Autodesk Fusion 360 part; units mm, degrees
sketch "Sketch1" plane through (0, 0, 0) normal (0, 0, 1) x (1, 0, 0)
  line L0 (19.05, -25.4) -> (-19.05, -25.4)
  line L1 (-19.05, -25.4) -> (-19.05, 25.4)
  line L2 (-19.05, 25.4) -> (19.05, 25.4)
  line L3 (19.05, 25.4) -> (19.05, -25.4)
  line L4 (19.05, -25.4) -> (-19.05, 25.4) construction
  line L5 (-19.05, -25.4) -> (19.05, 25.4) construction
  dimension "d1" = 38.1
  dimension "d2" = 50.8
extrude "Extrude1" add sketch "Sketch1" along normal blind 6.35
sketch "Sketch2" plane through (0, 0, 6.35) normal (0, 0, 1) x (-1, 0, 0)
  line L0 (-19.05, -25.4) -> (19.05, -25.4)
  line L1 (19.05, -25.4) -> (19.05, 25.4)
  line L2 (19.05, 25.4) -> (-19.05, 25.4)
  line L3 (-19.05, 25.4) -> (-19.05, -25.4)
  line L4 (19.05, -12.7) -> (3.81, -12.7)
  line L5 (3.81, -12.7) -> (3.81, 12.7)
  line L6 (3.81, 12.7) -> (19.05, 12.7)
  line L7 (19.05, 12.7) -> (19.05, -12.7)
  line L8 (-19.05, -15.24) -> (3.81, -15.24)
  line L9 (3.81, -15.24) -> (3.81, 15.24)
  line L10 (3.81, 15.24) -> (-19.05, 15.24)
  line L11 (-19.05, 15.24) -> (-19.05, -15.24)
  dimension "d5" = 15.24
  dimension "d6" = 25.4
  dimension "d7" = 12.7
  dimension "d9" = 10.16
  dimension "d14" = 10.16
extrude "Extrude2" add sketch "Sketch2" along normal blind 15.24 contours L1 L4 L5 L6 L7 L9
extrude "Extrude3" add sketch "Sketch2" along normal blind 29.21 contours L3 L5 L8 L9 L10 L11
sketch "Sketch3" plane through (0, -12.7, 0) normal (0, -1, 0) x (1, 0, 0)
  line L0 (-19.05, 6.35) -> (-3.81, 6.35)
  line L1 (-3.81, 6.35) -> (-3.81, 21.59)
  line L2 (-3.81, 21.59) -> (-19.05, 21.59)
  line L3 (-19.05, 21.59) -> (-19.05, 6.35)
  circle A0 centre (-11.43, 13.97) radius 3.937
  dimension "d15" = 7.874
  dimension "d16" = 7.62
  dimension "d17" = 7.62
extrude "Extrude4" cut sketch "Sketch3" against normal through all contours A0
fillet "Fillet1" radius 2.54 2 edges at (-19.05, -25.4, 3.175) (-19.05, 25.4, 3.175)
fillet "Fillet2" radius 1.27 6 edges at (1.27, 25.4, 6.35) (-18.3061, 24.6561, 6.35) (-19.05, 17.78, 6.35) (-19.05, -17.78, 6.35) (-18.3061, -24.6561, 6.35) (1.27, -25.4, 6.35)
fillet "Fillet3" radius 7.62 1 edges at (-19.05, 0, 21.59)
fillet "Fillet4" radius 1.27 14 edges at (-3.81, 15.24, 20.955) (7.62, 15.24, 35.56) (-3.81, 0, 35.56) (7.62, -15.24, 35.56) (-3.81, -15.24, 20.955) (19.05, 0, 35.56) (19.05, -15.24, 20.955) (19.05, 15.24, 20.955) (19.05, -25.4, 2.54) (19.05, -25.028, 5.978) (19.05, -19.685, 6.35) (19.05, 19.685, 6.35) (19.05, 25.028, 5.978) (19.05, 25.4, 2.54)
fillet "Fillet5" radius 0.508 6 edges at (-7.62, 12.7, 21.59) (-16.8182, 12.7, 19.3582) (-19.05, 12.7, 9.525) (-19.05, -12.7, 9.525) (-16.8182, -12.7, 19.3582) (-7.62, -12.7, 21.59)
sketch "Sketch4" plane through (0, 15.24, 0) normal (0, 1, 0) x (-1, 0, 0)
  line L0 (2.54, 6.35) -> (2.54, 34.29)
  line L1 (2.54, 34.29) -> (-17.78, 34.29)
  line L2 (-17.78, 34.29) -> (-17.78, 6.35)
  line L3 (-17.78, 6.35) -> (2.54, 6.35)
  line L4 (-13.97, 31.75) -> (-1.27, 31.75)
  line L5 (-1.27, 31.75) -> (-1.27, 21.59)
  line L6 (-1.27, 21.59) -> (-13.97, 21.59)
  line L7 (-13.97, 21.59) -> (-13.97, 31.75)
  dimension "d29" = 3.81
  dimension "d30" = 3.81
  dimension "d31" = 2.54
  dimension "d32" = 10.16
extrude "Extrude5" cut sketch "Sketch4" against normal through all contours L4 L5 L6 L7
sketch "Sketch5" plane through (-3.81, 0, 0) normal (-1, 0, 0) x (0, -1, 0)
  line L0 (13.97, 6.35) -> (13.97, 34.29)
  line L1 (13.97, 34.29) -> (-13.97, 34.29)
  line L2 (-13.97, 34.29) -> (-13.97, 6.35)
  line L3 (-13.97, 6.35) -> (-12.7, 6.35)
  line L4 (-12.7, 6.35) -> (-12.7, 21.082)
  arc A0 (-12.192, 21.59) -> (-12.7, 21.082) centre (-12.192, 21.082) ccw
  line L5 (-12.192, 21.59) -> (12.192, 21.59)
  arc A1 (12.7, 21.082) -> (12.192, 21.59) centre (12.192, 21.082) ccw
  line L6 (12.7, 21.082) -> (12.7, 6.35)
  line L7 (12.7, 6.35) -> (13.97, 6.35)
  line L8 (-11.43, 33.02) -> (11.43, 33.02)
  line L9 (11.43, 33.02) -> (11.43, 24.2438)
  line L10 (11.43, 24.2438) -> (-11.43, 24.2438)
  line L11 (-11.43, 24.2438) -> (-11.43, 33.02)
extrude "Extrude6" cut sketch "Sketch5" against normal up to surface (17.78 mm away) contours L8 L9 L10 L11
sketch "Sketch6" plane through (0, 0, 0) normal (0, 0, -1) x (1, 0, 0)
  arc A0 (19.05, 24.13) -> (17.78, 25.4) centre (17.78, 24.13) ccw
  line L0 (17.78, 25.4) -> (-16.51, 25.4)
  arc A1 (-16.51, 25.4) -> (-19.05, 22.86) centre (-16.51, 22.86) ccw
  line L1 (-19.05, 22.86) -> (-19.05, -22.86)
  arc A2 (-19.05, -22.86) -> (-16.51, -25.4) centre (-16.51, -22.86) ccw
  line L2 (-16.51, -25.4) -> (17.78, -25.4)
  arc A3 (17.78, -25.4) -> (19.05, -24.13) centre (17.78, -24.13) ccw
  line L3 (19.05, -24.13) -> (19.05, 24.13)
  circle A4 centre (0, 0) radius 3.5
  dimension "d36" = 7
extrude "Extrude7" cut sketch "Sketch6" against normal blind 2 contours A4
Source: CAD feature listing. Evaluate the final solid. Frame: model axes, mm. A direction names the side the tool comes from. Coordinates: 2 decimals unless noted, no trailing zeros. Loops run counter-clockwise (first coordinate to the right, second up) from the corner with the lowest first, then second, coordinate; pieces in that order, holes last. Notation, with made-up numbers: (-3.75, 11.5) -> (45.25, 11.5) arc R19 cw to (45.25, 37.5) -> close; hole circle Ø5 at (-39, 26.5). An arc over 180 degrees is marked (long way). One line per item, written item: value. Start each with the question number.
Q1. Line query: line 1 along Y through (x, z) = (0, 0.4); line 2 along Z through (x, y) = (10.5, -7); line 3 along Z through (x, y) = (-11.43, -6.25). Output: solid intervals per line, ascending.
Q2. Section query B-B, the plane y = -8. Return the cut outline in (x, z), and give its area (3 significant figures).
Q3. Set-up query: faces 4 (the face through (-10, 12.7, 10)), 5 (the face through (18.668, -14.878, 19.889)), 6 (the face through (7, -15.24, 20)), 7 (the face through (18.688, 18.979, 5.968)). Return all of +Z, -Z, +X, -X, +Y, -Y with unobstructed straight access to the full face (end or side cutting, diameter ignored); none if empty.
Q4. Section query C-C, the plane z = 7. Return the cut outline in (x, y), and give its area (3 significant figures).
Q5. Contact query for flat-ended pins moving along their axis: P1, Ø12, axis at x = -11, z = 14.5, coming from the -Y side; P2, Ø12, axis at x = 7.5, z = 17, coming from the +Y side; P3, Ø6, axis at x = -7, y = 2.5, coming from the +Z side. Output: stop coordinate, or through.
Q6. Mould query, pull axis X, two halves, no side actions, for faces 1 (the face through (8, 13, 31.75)), 2 (the face through (18.668, 0.196, 35.198)), 3 (the face through (-3.81, 2, 23)). Classes: pulls with the +X half, pulls with the -X half, needs draft (parallel to the pull), parting line crosses it, or undercut.
Q7. Section query A-A, the plane x = 9. Return the cut outline in (y, z), and give its area (3 significant figures).
Q8. Section query D-D, the plane x = 0. Return the cut outline in (y, z).
Results:
1. line 1: -25.4 to -3.5, 3.5 to 25.4
1. line 2: 0 to 21.59, 33.02 to 35.56
1. line 3: 0 to 10.03, 17.91 to 21.59
2. outline: (-19.05, 0) -> (19.05, 0) -> (19.05, 34.29) arc R1.27 ccw to (17.78, 35.56) -> (-2.54, 35.56) arc R1.27 ccw to (-3.81, 34.29) -> (-3.81, 33.02) -> (13.97, 33.02) -> (13.97, 21.59) -> (1.27, 21.59) -> (1.27, 24.24) -> (-3.81, 24.24) -> (-3.81, 21.59) -> (-11.43, 21.59) arc R7.62 ccw to (-19.05, 13.97) -> close; hole circle Ø7.87 at (-11.43, 13.97)
2. area: 890 mm^2
3. face 4: +Z, -X, +Y
3. face 5: +Z, +X, -Y
3. face 6: +Z, +X, -X, -Y
3. face 7: +Z, +X, +Y
4. outline: (-19.05, -12.19) arc R0.51 ccw to (-18.54, -12.7) -> (-3.81, -12.7) -> (-3.81, -13.97) arc R1.27 ccw to (-2.54, -15.24) -> (17.78, -15.24) arc R1.27 ccw to (19.05, -13.97) -> (19.05, 13.97) arc R1.27 ccw to (17.78, 15.24) -> (-2.54, 15.24) arc R1.27 ccw to (-3.81, 13.97) -> (-3.81, 12.7) -> (-18.54, 12.7) arc R0.51 ccw to (-19.05, 12.19) -> close
4. area: 1,080 mm^2
5. P1: y = -12.7
5. P2: y = 15.24
5. P3: z = 21.59
6. face 1: undercut
6. face 2: pulls with the +X half
6. face 3: pulls with the -X half
7. outline: (-25.4, 0) -> (25.4, 0) -> (25.4, 5.08) arc R1.27 ccw to (24.13, 6.35) -> (15.24, 6.35) -> (15.24, 21.59) -> (-15.24, 21.59) -> (-15.24, 6.35) -> (-24.13, 6.35) arc R1.27 ccw to (-25.4, 5.08) -> close; (-15.24, 31.75) -> (-11.43, 31.75) -> (-11.43, 33.02) -> (11.43, 33.02) -> (11.43, 31.75) -> (15.24, 31.75) -> (15.24, 34.29) arc R1.27 ccw to (13.97, 35.56) -> (-13.97, 35.56) arc R1.27 ccw to (-15.24, 34.29) -> close
7. area: 873 mm^2
8. outline: (-25.4, 0) -> (-3.5, 0) -> (-3.5, 2) -> (3.5, 2) -> (3.5, 0) -> (25.4, 0) -> (25.4, 5.08) arc R1.27 ccw to (24.13, 6.35) -> (15.24, 6.35) -> (15.24, 34.29) arc R1.27 ccw to (13.97, 35.56) -> (-13.97, 35.56) arc R1.27 ccw to (-15.24, 34.29) -> (-15.24, 6.35) -> (-24.13, 6.35) arc R1.27 ccw to (-25.4, 5.08) -> close; hole (-11.43, 24.24) -> (11.43, 24.24) -> (11.43, 33.02) -> (-11.43, 33.02) -> close
